The listing builds one solid part. Answer for the finished solid, in the listing's coordinates (mm). A direction names the side the tool comes from. Give positions to 0.01 mm unless a question says otherwise; leave off trailing zeros. Write each loop counter-clockwise with the first axis right and the second up, starting at its lowest first coordinate (ties: lowest second). Pieces come first, ordered by that corner, then holes. Notation, with made-up numbers: (-12.5, -23) - (36.5, -23) arc R7 ccw to (36.5, -17) - close; hole circle Ø10 at (29.5, 66). An arc over 180 degrees is marked (long way). One line per question, with ' | ' between items. Start each with the question number.
1. A cutting plane is placed at B-B (x = -7). Determine the outline of the cut face in (y, z), then the cut area to 3 significant figures.
2. Find the intervals of material crossed by L1, parallel to Y at x = 16.65, z = 0; L2, parallel to X at y = -6, z = -8.5; L3, parallel to X at y = 6, z = -7, in increasing order. Write a range as from..to.
3. The mould has two halves that part along X. Classify faces 4 (the face through (25.084, -3.486, -3.585)), 5 (the face through (19, 0, 6)), 6 (the face through (28.659, 9.274, -2.059)): +X half, -X half, draft (parallel to the pull), parting line (faces both ways), or undercut.
4. Given P1, Ø1, axis at y = 9, z = -7, coming from the +X side; P2, Ø3, axis at x = -6, y = 2.5, coming from the -Z side; P3, Ø1.1, axis at y = 0.5, z = 4.5, coming from the +X side, each flat-ended and moving along its own axis, determine where each tip first touches the part or whether it passes through.
5. For faces 1 (the face through (28, 4, 9)), 2 (the face through (-13, -2, 0)), 3 (the face through (25.084, 3.486, 3.585)), determine the directions among +Z, -Z, +X, -X, +Y, -Y from which every point of the face is accessible in a straight line to the end or side of a thin tool.
6. A cutting plane is placed at A-A (z = 16.5). Determine the outline of the cut face in (x, y), then the cut area to 3 significant figures.
```python
from build123d import *

# Parameters (mm, degrees)
PER_AGE5_D              = 10
PER_AGE5_DEPTH          = 17
PER_AGE5_TIP            = 3.004303095
ENL_V_MAT_EXTRU_1_DEPTH = 12


with BuildPart() as part:
    # Esquisse1 → Base-Révolution (revolve)
    with BuildSketch(Plane.XY, mode=Mode.PRIVATE) as base_r_volution_sk:
        Polygon((0, 0), (0, 18.5), (5, 18.5), (5, 9), (7, 9), (7, 10), (28, 10), (28, 9.5), (29.3, 9.5), (29.3, 10), (30, 10), (31, 9), (31, 0), align=None)
    revolve(base_r_volution_sk.sketch.rotate(Axis((0, 0, 0), (1, 0, 0)), 90), axis=Axis((0, 0, 0), (1, 0, 0)))

    # Esquisse2 → Boss.-Révol.1 (revolve)
    with BuildSketch(Plane.XY):
        Polygon((-26, 5), (-26, 11), (-25, 12), (-2, 12), (-2, 11), (0, 11), (0, 5), align=None)
    revolve(axis=Axis((0, 5, 0), (-1, 0, 0)))

    # Perçage5
    with Locations(Plane(origin=(31, 0, 0), x_dir=(0, 0, -1), z_dir=(1, 0, 0))):
        with Locations((0, 0)):
            Hole(PER_AGE5_D / 2, depth=PER_AGE5_DEPTH)
            with Locations((0, 0, -(PER_AGE5_DEPTH + PER_AGE5_TIP / 2))):  # 118° drill point
                Cone(0, PER_AGE5_D / 2, PER_AGE5_TIP, mode=Mode.SUBTRACT)

    # Esquisse5 → Enlèv. mat.-Extru.1 (cut)
    with BuildSketch(Plane(origin=(31, 0.918663762, 3.195352215), x_dir=(0, 0, -1), z_dir=(1, 0, 0))):
        Polygon((-3.875715597, -0.918663762), (3.195352215, 6.15240405), (10.266420027, -0.918663762), (3.195352215, -7.989731574), align=None)
    extrude(amount=-ENL_V_MAT_EXTRU_1_DEPTH, mode=Mode.SUBTRACT)


solid = part.part
```
Determined:
1) outline: circle Ø14 at (5, 0) | area: 154 mm2
2) L1: -10..-5, 5..10 | L2: 0..5 | L3: 0..5, 7..30.78
3) face 4: draft | face 5: +X half | face 6: undercut
4) P1: x = 5 | P2: z = -6.93 | P3: x = 19
5) face 1: none | face 2: -X | face 3: +X
6) outline: (0, -8.37) - (5, -8.37) - (5, 8.37) - (0, 8.37) - close | area: 83.7 mm2
